CAD build for the part. Positions are in the model's coordinates, mm. Round coordinates to 2 decimals unless told otherwise and drop trailing zeros. Order: outer loops, then holes, each group sorted by start corner. A loop starts at its lowest first (then second) coordinate and runs counter-clockwise, first axis right, second up. Notation, with made-up numbers: (-33, 16.25) - (23, 16.25) arc R10 cw to (23, 28.25) - close; hole circle Ø4 at (43.25, -21). An arc over 180 degrees is marked (long way). Use one line per item in the form item = value. Start each with the question number.
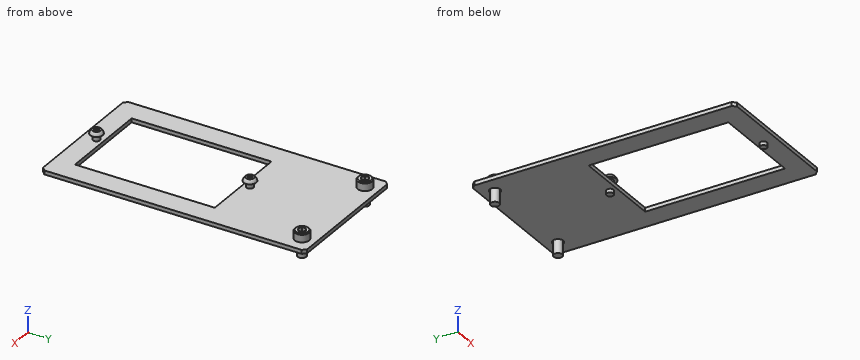
from build123d import *

# Parameters (mm, degrees)
SKETCH1_W                = 80
SKETCH1_H                = 155
BOSS_EXTRUDE1_DEPTH      = 2.3
SKETCH2_R                = 3.1
SKETCH2_W                = 54
SKETCH2_H                = 82
CUT_EXTRUDE1_DEPTH       = 153.362364119
CHAMFER1_SIZE            = 2
CUT_EXTRUDE2_DEPTH       = 2.5
CHAMFER2_SIZE            = 0.6
CHAMFER2_OF_MIRROR1_SIZE = 0.6
CUT_EXTRUDE3_DEPTH       = 1.3
LPATTERN1_COUNT          = 2
LPATTERN1_PITCH          = 90


with BuildPart() as part:
    # Sketch1 → Boss-Extrude1 (new body)
    with BuildSketch(Plane.XY):
        with Locations((0, -69.5)):
            Rectangle(SKETCH1_W, SKETCH1_H)
    extrude(amount=BOSS_EXTRUDE1_DEPTH)

    # Sketch2 → Cut-Extrude1 (cut, through all)
    with BuildSketch(Plane.XY.offset(2.3)):
        with Locations((-30, 0)):
            Circle(SKETCH2_R)
        with Locations((30, 0)):
            Circle(SKETCH2_R)
        with Locations((0, -94)):
            Rectangle(SKETCH2_W, SKETCH2_H)
    extrude(amount=-CUT_EXTRUDE1_DEPTH, mode=Mode.SUBTRACT)

    # Chamfer1
    chamfer1_edges = [part.edges().sort_by_distance(p)[0] for p in [
        (40, -147, 1.15),
        (40, 8, 1.15),
        (-40, 8, 1.15),
        (-40, -147, 1.15),
    ]]
    chamfer(chamfer1_edges, length=CHAMFER1_SIZE)

    # Sketch3 → Revolve1 (revolve)
    with BuildSketch(Plane(origin=(0, 0, 0), x_dir=(1, 0, 0), z_dir=(0, 1, 0))):
        Polygon((-28, -7.3), (-25.75, -7.3), (-25.75, -2.3), (-27.5, -2.3), (-27.5, 7.7), (-30, 7.7), (-30, -4.264101615), (-28, -4.8), align=None)
    revolve1 = revolve(axis=Axis((-30, 0, 7.3), (0, 0, -1)))

    # Sketch4 → Cut-Extrude2 (cut)
    with BuildSketch(Plane.XY.offset(7.3)):
        Polygon((-30, 2.309401077), (-32, 1.154700538), (-32, -1.154700538), (-30, -2.309401077), (-28, -1.154700538), (-28, 1.154700538), align=None)
    cut_extrude2 = extrude(amount=-CUT_EXTRUDE2_DEPTH, mode=Mode.SUBTRACT)

    # Chamfer2
    chamfer2_edges = [part.edges().sort_by_distance(p)[0] for p in [
        (-34.25, 0, 7.3),
    ]]
    chamfer(chamfer2_edges, length=CHAMFER2_SIZE)

    # Mirror1: Revolve1, Cut-Extrude2 across plane
    add(revolve1.mirror(Plane(origin=(0, 0, 0), x_dir=(0, 0, 1), z_dir=(1, 0, 0))))
    add(cut_extrude2.mirror(Plane(origin=(0, 0, 0), x_dir=(0, 0, 1), z_dir=(1, 0, 0))), mode=Mode.SUBTRACT)

    # Chamfer2 of Mirror1
    chamfer2_of_mirror1_edges = [part.edges().sort_by_distance(p)[0] for p in [
        (34.25, 0, 7.3),
    ]]
    chamfer(chamfer2_of_mirror1_edges, length=CHAMFER2_OF_MIRROR1_SIZE)

    # Sketch5 → Revolve2 (revolve)
    with BuildSketch(Plane(origin=(0, 0, 0), x_dir=(0, 0, -1), z_dir=(1, 0, 0)), mode=Mode.PRIVATE) as revolve2_sk:
        with BuildLine():
            Line((2.2, -47), (-5.8, -47))
            Line((-5.8, -47), (-5.8, -45.265030121))
            ThreePointArc((-5.8, -45.265030121), (-7.010286128, -45.715063637), (-8, -46.544394168))
            Line((-8, -46.544394168), (-8, -47.75))
            Line((-8, -47.75), (-6.7, -47.75))
            Line((-6.7, -47.75), (-5.978312164, -49))
            Line((-5.978312164, -49), (2.2, -49))
            Line((2.2, -49), (2.2, -47))
        make_face()
    revolve2 = revolve(revolve2_sk.sketch.rotate(Axis((0, -49, 8), (0, 0, -1)), 90), axis=Axis((0, -49, 8), (0, 0, -1)))

    # Sketch6 → Cut-Extrude3 (cut)
    with BuildSketch(Plane.XY.offset(8)):
        Polygon((0, -47.556624327), (-1.25, -48.278312164), (-1.25, -49.721687836), (0, -50.443375673), (1.25, -49.721687836), (1.25, -48.278312164), align=None)
    cut_extrude3 = extrude(amount=-CUT_EXTRUDE3_DEPTH, mode=Mode.SUBTRACT)

    # LPattern1: Revolve2, Cut-Extrude3 ×2
    with Locations(*[(0, -i * LPATTERN1_PITCH, 0) for i in range(1, LPATTERN1_COUNT)]):
        add(revolve2)
        add(cut_extrude3, mode=Mode.SUBTRACT)


solid = part.part
(1) Wall check: line 1 (Y direction, x = 30, z = 1.05); line 2 (Y direction, x = -28.5, z = -0.25); line 3 (Z direction, x = 6.5, y = -12). Give the ranges that are in metal, low to high. Write a range as [from, to].
(2) Slice it at B-B (x = 13). Give the cut face in (y, z), and give its area (3 significant figures).
(3) Slice it at C-C (z = -4). Give the cut face in (x, y).
(4) Slice it at A-A (y = -68.5). Give the cut face in (x, z), and give its area (3 significant figures).
(5) Slice it at D-D (y = -30.5). Give the cut face in (x, z).
(6) Flat gauge pins, fed straight in: P1, Ø0.5, axis at x = 31.5, y = -1, coming from the +Z side; P2, Ø1.5, axis at x = 29.5, y = -114.5, coming from the +Z side; P3, Ø4.5, axis at x = -0.5, y = -48.5, coming from the -Z side. Where does each tip first touch, or does it go through?
Results list:
q1.line_1 = [-147, -3.1], [-2.5, 2.5], [3.1, 8]
q1.line_2 = [-2, 2]
q1.line_3 = [0, 2.3]
q2.outline = (-147, 0) - (-135, 0) - (-135, 2.3) - (-147, 2.3) - close; (-53, 0) - (8, 0) - (8, 2.3) - (-53, 2.3) - close
q2.area = 168 mm²
q3.outline = circle Ø5 at (-30, 0); circle Ø5 at (30, 0)
q4.outline = (-40, 0) - (-27, 0) - (-27, 2.3) - (-40, 2.3) - close; (27, 0) - (40, 0) - (40, 2.3) - (27, 2.3) - close
q4.area = 59.8 mm²
q5.outline = (-40, 0) - (40, 0) - (40, 2.3) - (-40, 2.3) - close
q6.P1 = 4.8
q6.P2 = 2.3
q6.P3 = -2.2
